Work out the finished part from the listing and answer in its coordinate system (mm). Give positions to 0.01 mm unless a question says otherwise; leave off trailing zeros. Loops run counter-clockwise (first coordinate to the right, second up) from the corner with the lowest first, then second, coordinate; pieces in that order, holes last. Notation, with made-up numbers: (35.5, 4) - (87.5, 4) arc R22 cw to (87.5, 36) - close; hole circle Ø10 at (64.25, 13.25). An arc over 180 degrees is marked (long way). Use CSV: the item, a comma, the result in double quotes.
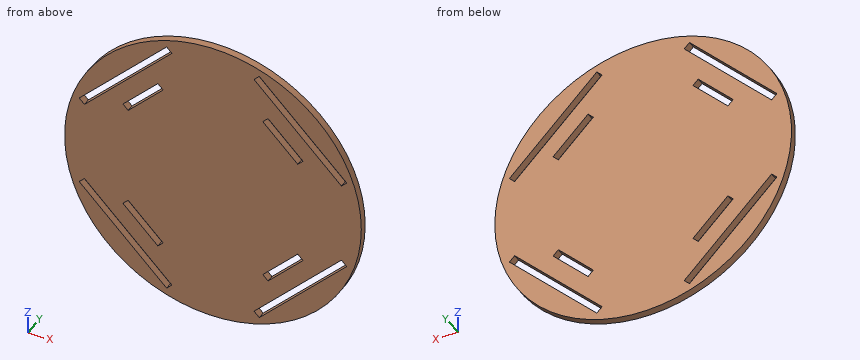
from build123d import *

# Parameters (mm, degrees)
SKETCH1_R           = 60
BOSS_EXTRUDE1_DEPTH = 1.5
CUT_EXTRUDE3_START  = -4
CUT_EXTRUDE3_DEPTH  = 5
CIRPATTERN1_COUNT   = 4
CUT_EXTRUDE4_DEPTH  = 4
CIRPATTERN2_COUNT   = 4


with BuildPart() as part:
    # Sketch1 → Boss-Extrude1 (new body, symmetric)
    with BuildSketch(Plane(origin=(0, 0, 0), x_dir=(1, 0, 0), z_dir=(0, 1, 0))):
        Circle(SKETCH1_R)
    extrude(amount=BOSS_EXTRUDE1_DEPTH, both=True)

    # Sketch4 → Cut-Extrude3 (cut)
    with BuildSketch(Plane(origin=(0, 1.5, 0), x_dir=(1, 0, 0), z_dir=(0, 1, 0)).offset(CUT_EXTRUDE3_START)):
        Polygon((16.617009358, 51.972348417), (51.972348417, 16.617009358), (54.093668761, 18.738329701), (18.738329701, 54.093668761), align=None)
    cut_extrude3 = extrude(amount=CUT_EXTRUDE3_DEPTH, mode=Mode.SUBTRACT)

    # CirPattern1: Cut-Extrude3 ×4 about axis
    cirpattern1_axis = Axis((0, 0, 0), (0, 1, 0))
    for i in range(1, CIRPATTERN1_COUNT):
        add(cut_extrude3.rotate(cirpattern1_axis, i * 360 / CIRPATTERN1_COUNT), mode=Mode.SUBTRACT)

    # Sketch5 → Cut-Extrude4 (cut, through all)
    with BuildSketch(Plane(origin=(0, 1.5, 0), x_dir=(1, 0, 0), z_dir=(0, 1, 0))):
        Polygon((22.273863607, 36.415999231), (36.415999231, 22.273863607), (34.294678888, 20.152543264), (20.152543264, 34.294678888), align=None)
    cut_extrude4 = extrude(amount=-CUT_EXTRUDE4_DEPTH, mode=Mode.SUBTRACT)

    # CirPattern2: Cut-Extrude4 ×4 about axis
    cirpattern2_axis = Axis((0, 0, 0), (0, 1, 0))
    for i in range(1, CIRPATTERN2_COUNT):
        add(cut_extrude4.rotate(cirpattern2_axis, i * 360 / CIRPATTERN2_COUNT), mode=Mode.SUBTRACT)


solid = part.part
Item 1: A cutting plane is placed at C-C on x = 46.5. Determine the outline of the cut face in (y, z), and give its area (3 significant figures).
Determined:
outline,"(-1.5, -37.92) - (1.5, -37.92) - (1.5, -26.33) - (-1.5, -26.33) - close; (-1.5, -22.09) - (1.5, -22.09) - (1.5, 22.09) - (-1.5, 22.09) - close; (-1.5, 26.33) - (1.5, 26.33) - (1.5, 37.92) - (-1.5, 37.92) - close"
area,"202 mm²"
Item 2: A cutting plane is placed at A-A on z = 50. Determine the outline of the cut face in (x, y).
Determined:
outline,"(-33.17, -1.5) - (-22.83, -1.5) - (-22.83, 1.5) - (-33.17, 1.5) - close; (-18.59, -1.5) - (18.59, -1.5) - (18.59, 1.5) - (-18.59, 1.5) - close; (22.83, -1.5) - (33.17, -1.5) - (33.17, 1.5) - (22.83, 1.5) - close"
Item 3: A cutting plane is placed at B-B on y = 0.8. State how many separate pieces and enclosed holes the cut face has, and give its area (3 significant figures).
Determined:
separate pieces,"1"
enclosed holes,"8"
area,"10,500 mm²"
Item 4: Find the intervals of material crossed by line 1 (X direction, y = 0.35, z = 18.5); line 2 (X direction, y = 0.15, z = -50); line 3 (Z direction, x = -33.5, y = 1.15), in increasing order.
Determined:
line 1,"x = -57.08 to -53.86, -50.09 to 50.09, 53.86 to 57.08"
line 2,"x = -33.17 to -22.83, -18.59 to 18.59, 22.83 to 33.17"
line 3,"z = -49.78 to -39.33, -35.09 to -25.19, -20.95 to 20.95, 25.19 to 35.09, 39.33 to 49.78"
Item 5: Given P1, Ø1, axis at x = -23, y = 0.5, coming from the -Z side, flat-ended and moving along its own axis, determine where the tip first touches the part or whether it passes through.
Determined:
P1,"stops at z = -55.62"
Item 6: A cutting plane is placed at D-D on x = -10.5. Determine the outline of the cut face in (y, z), and give its area (3 significant figures).
Determined:
outline,"(-1.5, -59.07) - (1.5, -59.07) - (1.5, 59.07) - (-1.5, 59.07) - close"
area,"354 mm²"
